Answer from the drawing. Dimensions are ordinates in mm from the lowest x, y and z of the part. A direction names the side the tool comes from. Round coordinates to 2 decimals unless told otherwise and drop trailing zeros. Write each loop counter-clockwise with the first axis right and the second up, starting at its lowest first coordinate (ties: lowest second). Pieces come first, ordered by that corner, then holes.
1. A tool of negligible diameter and unlimited length cuts with its end or side. For the marked faces 1 and 2, from which of +Z, -Z, +X, -X, +Y, -Y can it reach the whole face along a straight path? Write none if from no direction.
2. Straight lines are drawn through the part: probe 1 along X at (y, z) = (2.45, 15); probe 2 along Y at (x, z) = (18.75, 12.75). For each, find the intervals that lie inside material, in ascending order.
3. Find section D-D (x = 7.75). Write down the section's boundary in (y, z), and give its area (3 significant figures).
4. Find section A-A (x = 15). Write down the section's boundary in (y, z), and give its area (3 significant figures).
5. Find section B-B (z = 15). Write down the section's boundary in (x, y), and give its area (3 significant figures).
6. Flat-ended cylindrical pins translate along their axes: pin 1 Ø12 at (y, z) = (9.5, 9.5) entering from +X; pin 2 Ø8 at (x, z) = (8.5, 23) entering from +Y. Find the tip coordinate at first contact, or state that the pin passes through.
7. Find section C-C (z = 4). Write down the section's boundary in (x, y).
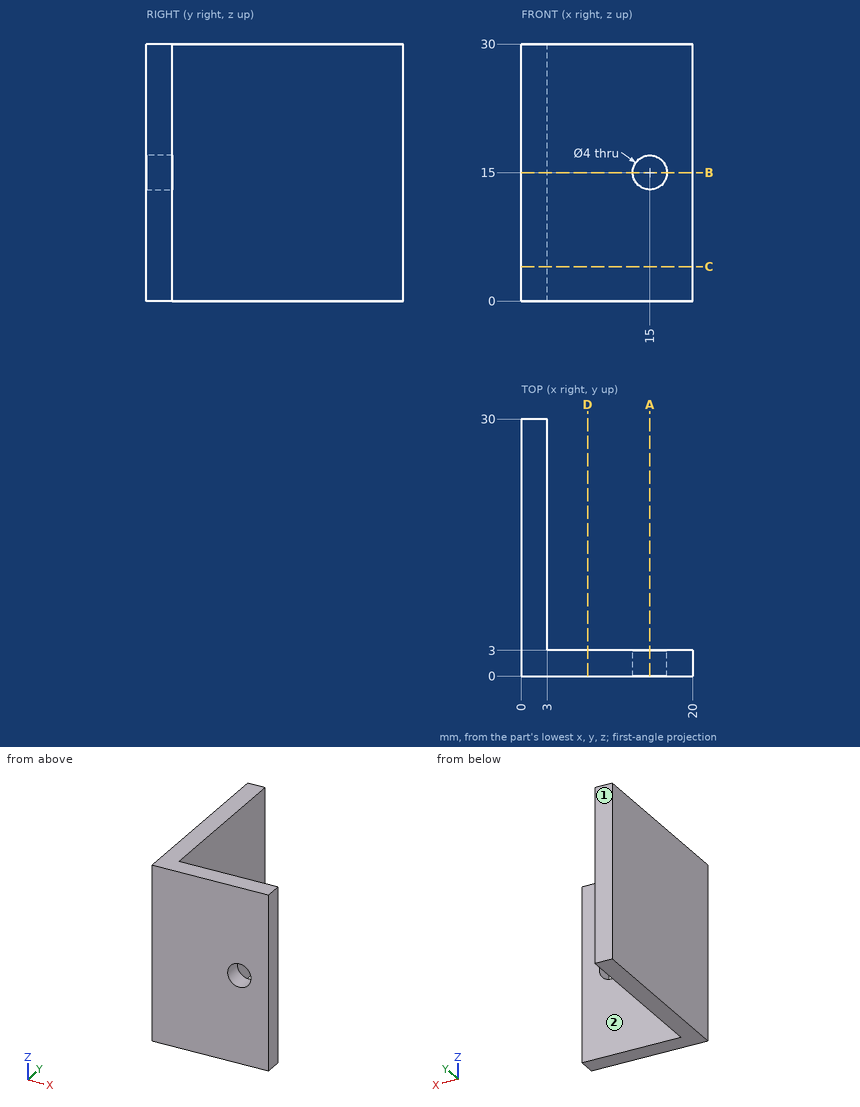
Worked answers:
1. face 1: +Z, -Z, +X, -X, +Y
1. face 2: +Z, -Z, +X, +Y
2. probe 1: x = 0 to 13, 17 to 20
2. probe 2: y = 0 to 3
3. outline: (0, 0) - (3, 0) - (3, 30) - (0, 30) - close
3. area: 90.0 mm2
4. outline: (0, 0) - (3, 0) - (3, 13) - (0, 13) - close; (0, 17) - (3, 17) - (3, 30) - (0, 30) - close
4. area: 78.0 mm2
5. outline: (0, 0) - (13, 0) - (13, 3) - (3, 3) - (3, 30) - (0, 30) - close; (17, 0) - (20, 0) - (20, 3) - (17, 3) - close
5. area: 129 mm2
6. pin 1: stops at x = 3
6. pin 2: stops at y = 3
7. outline: (0, 0) - (20, 0) - (20, 3) - (3, 3) - (3, 30) - (0, 30) - close
